The model under review builds one solid part; all positions refer to its coordinate system, in mm. Face numbers are marked on the shaded views. A direction names the side the tool comes from. Round coordinates to 2 decimals unless told otherwise and drop trailing zeros. Loops run counter-clockwise (first coordinate to the right, second up) from the corner with the lowest first, then second, coordinate; pieces in that order, holes last. Notation, with made-up numbers: M -33,16 L 5,16 A14 ccw 5,33 Z; hole C 87,6.5 d1. An arc over 180 degrees is marked long. Use a Markdown table: item, result. Add a question column.
```python
from build123d import *

# Parameters (mm, degrees)
F0_R     = 9
F0_W     = 10
F0_H     = 10
F0_W_2   = 8.2
F0_H_2   = 8.2
F1_DEPTH = 2
F2_DEPTH = 20
F3_SIZE  = 0.5


with BuildPart() as f1:
    # F0 (on Top) → F1 (new body)
    with BuildSketch(Plane.XY):
        Circle(F0_R)
        Rectangle(F0_W, F0_H, mode=Mode.SUBTRACT)
        Rectangle(F0_W, F0_H)
        Rectangle(F0_W_2, F0_H_2, mode=Mode.SUBTRACT)
    extrude(amount=F1_DEPTH)

    # F0 (on Top) → F2 (join)
    with BuildSketch(Plane.XY):
        Rectangle(F0_W, F0_H)
        Rectangle(F0_W_2, F0_H_2, mode=Mode.SUBTRACT)
    extrude(amount=F2_DEPTH)

    # F3
    f3_edges = [f1.edges().sort_by_distance(p)[0] for p in [
        (0, -5, 20),
        (5, 0, 20),
        (0, 5, 20),
        (-5, 0, 20),
    ]]
    chamfer(f3_edges, length=F3_SIZE)


solid = f1.part
```
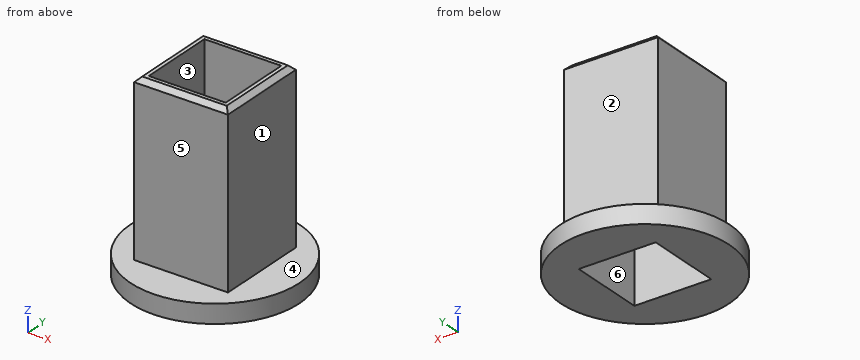
(1) Consider section C-C, the plane z = 6. Give the boundary of the cut face in (x, y), then the cut area to 3 significant figures.
(2) To check wall thickness, follow probe 1 along X at (y, z) = (-3.75, 2.75); probe 2 along Y at (x, z) = (4.25, 2.75). State the ranges of each line that lie inside material, in increasing order.
(3) Draft analysis for pull direction X (two halves, no side actions). For the marked faces 1, 2 and 3, state which applies: released by +X, released by -X, zero draft, split by the parting line, or undercut.
(4) Consider section A-A, the plane y = 0. Give the boundary of the cut face in (x, z).
(5) Consider section D-D, the plane x = 7.5. Give the boundary of the cut face in (y, z), then the cut area to 3 significant figures.
(6) For the marked faces 4, 5 and 6, list the 3-axis set-ups (+Z, -Z, +X, -X, +Y, -Y) from which the entire face can be reached by the end or side of a thin tool; tool diameter is ignored.
(7) Insertion check: pin 1 Ø3 at (x, y) = (4.5, 2) entering from -Z; pin 2 Ø9 at (y, z) = (1, 10) entering from -X; pin 3 Ø9 at (x, z) = (0.5, 9.5) entering from -Y; pin 4 Ø4 at (y, z) = (-2, 9.5) entering from +X. Each pin has a flat end and moves straight along its axis. Give the tip position at first contact, or say it passes through.
Found:
| question | item | result |
|---|---|---|
| 1 | outline | M -5,-5 L 5,-5 L 5,5 L -5,5 Z; hole M -4.1,-4.1 L 4.1,-4.1 L 4.1,4.1 L -4.1,4.1 Z |
| 1 | area | 32.8 mm^2 |
| 2 | probe 1 | x = -5 to -4.1, 4.1 to 5 |
| 2 | probe 2 | y = -5 to 5 |
| 3 | face 1 | released by +X |
| 3 | face 2 | zero draft |
| 3 | face 3 | undercut |
| 4 | outline | M -9,0 L -4.1,0 L -4.1,20 L -4.5,20 L -5,19.5 L -5,2 L -9,2 Z; M 4.1,0 L 9,0 L 9,2 L 5,2 L 5,19.5 L 4.5,20 L 4.1,20 Z |
| 5 | outline | M -4.97,0 L 4.97,0 L 4.97,2 L -4.97,2 Z |
| 5 | area | 19.9 mm^2 |
| 6 | face 4 | +Z |
| 6 | face 5 | +Z, +X, -X, -Y |
| 6 | face 6 | +Z, -Z |
| 7 | pin 1 | stops at z = 0 |
| 7 | pin 2 | stops at x = -5 |
| 7 | pin 3 | stops at y = -5 |
| 7 | pin 4 | stops at x = 5 |
